```python
from build123d import *

# Parameters (mm, degrees)
F_1_8_0_125_DIAMETER_HOLE1_D     = 3.175
F_1_8_0_125_DIAMETER_HOLE1_DEPTH = 12.954
F_1_8_0_125_DIAMETER_HOLE1_TIP   = 0.953866233
F_6_32_TAPPED_HOLE1_D            = 2.7051
F_6_32_TAPPED_HOLE1_DEPTH        = 6.349
F_6_32_TAPPED_HOLE1_TIP          = 0.81269403
FILLET1_R                        = 0.635
CUT_EXTRUDE1_DEPTH               = 0.0254


with BuildPart() as part:
    # Sketch1 → Revolve1 (revolve)
    with BuildSketch(Plane.XY):
        Polygon((0, 15.875), (6.35, 15.875), (6.35, 3.683), (5.715, 3.048), (5.715, 0), (4.7625, 0), (4.7625, 3.9878), (0, 3.9878), align=None)
    revolve(axis=Axis((0, 0, 0), (0, 1, 0)))

    # 1/8 (0.125) Diameter Hole1
    with Locations(Plane(origin=(0, 0, 0), x_dir=(-1, 0, 0), z_dir=(0, -1, 0))):
        with Locations((0, 0)):
            Hole(F_1_8_0_125_DIAMETER_HOLE1_D / 2, depth=F_1_8_0_125_DIAMETER_HOLE1_DEPTH)
            with Locations((0, 0, -(F_1_8_0_125_DIAMETER_HOLE1_DEPTH + F_1_8_0_125_DIAMETER_HOLE1_TIP / 2))):  # 118° drill point
                Cone(0, F_1_8_0_125_DIAMETER_HOLE1_D / 2, F_1_8_0_125_DIAMETER_HOLE1_TIP, mode=Mode.SUBTRACT)

    # #6-32 Tapped Hole1
    with Locations(Plane(origin=(0, 0, -6.35), x_dir=(-1, 0, 0), z_dir=(0, 0, -1))):
        with Locations((0, 7.239)):
            Hole(F_6_32_TAPPED_HOLE1_D / 2, depth=F_6_32_TAPPED_HOLE1_DEPTH)
            with Locations((0, 0, -(F_6_32_TAPPED_HOLE1_DEPTH + F_6_32_TAPPED_HOLE1_TIP / 2))):  # 118° drill point
                Cone(0, F_6_32_TAPPED_HOLE1_D / 2, F_6_32_TAPPED_HOLE1_TIP, mode=Mode.SUBTRACT)

    # Fillet1
    fillet1_edges = [part.edges().sort_by_distance(p)[0] for p in [
        (-6.35, 15.875, 0),
    ]]
    fillet(fillet1_edges, radius=FILLET1_R)

    # Sketch6 → Cut-Extrude1 (cut)
    with BuildSketch(Plane(origin=(0, 15.875, 0), x_dir=(1, 0, 0), z_dir=(0, 1, 0))):
        Polygon((0, -5.334), (-0.762, -4.014177285), (0.762, -4.014177285), align=None)
    extrude(amount=-CUT_EXTRUDE1_DEPTH, mode=Mode.SUBTRACT)


solid = part.part
```
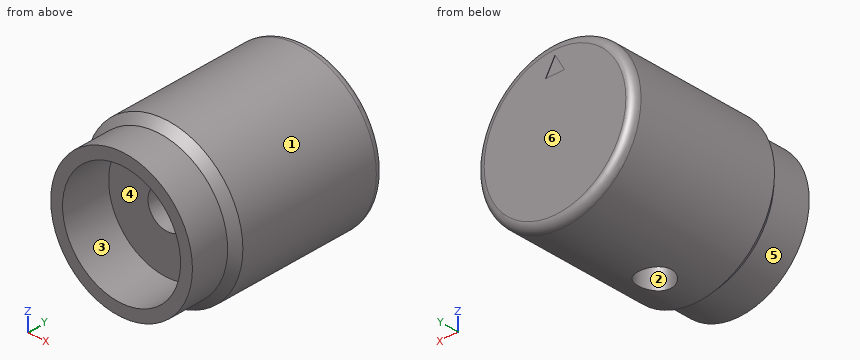
Source: CAD feature listing. Evaluate the final solid. Frame: model axes, mm. Face numbers are marked on the shaded views. A direction names the side the tool comes from. Round coordinates to 2 decimals unless told otherwise and drop trailing zeros. Loops run counter-clockwise (first coordinate to the right, second up) from the corner with the lowest first, then second, coordinate; pieces in that order, holes last. Notation, with made-up numbers: M 85.5,40.5 L 139.5,40.5 A13 cw 139.5,50.5 Z; hole C 59.25,18.25 d4. An arc over 180 degrees is marked long. Put each result on its own line as item: value.
(1) Pull-direction query (Z, two-part tool) for the marked faces 4, 5 and 6; classes: released by +Z, released by -Z, zero draft, split by the parting line, or undercut.
Solutions:
face 4: undercut
face 5: split by the parting line
face 6: zero draft
(2) Ray query, line 1 (X direction, y = 2.25, z = 0) (1 decimal); line 2 (Y direction, x = 0, z = -4.9) (3 decimals). Return the intervals inside material, ascending. Write a range as [from, to].
Solutions:
line 1: [-5.7, -4.8], [4.8, 5.7]
line 2: [0, 5.886], [8.592, 15.875]
(3) Access query for the marked faces 1, 2 and 3. Directions: +Z, -Z, +X, -X, +Y, -Y. A direction counts if a zero-diameter tool reaches every point of the face in a straight line with its end or side. Return the directions, or none.
Solutions:
face 1: +Y, -Y
face 2: -Z
face 3: -Y
(4) First-contact query: pin 1 (3 mm diameter, centred on x = -3.5, y = 9, fed in from +Z); pin 2 (3.5 mm diameter, centred on x = 0, z = 0, fed in from -Y); pin 3 (2 mm diameter, centred on x = 0, y = 7.239, fed in from -Z). Flat tips, straight axial feed; report the tip coordinate or a pass-through.
Solutions:
pin 1: z = 6.03
pin 2: y = 3.99
pin 3: z = 1.23
(5) Section A-A, the plane y = 14.5. Return loops of the section in (x, z), and give its area (3 significant figures).
Solutions:
outline: C 0,0 d12.7
area: 127 mm²
(6) Section B-B, the plane y = 1.5. Return loops of the section in (x, z) (1 decimal), and give its area (3 significant figures).
Solutions:
outline: C 0,0 d11.4; hole C 0,0 d9.5
area: 31.4 mm²
